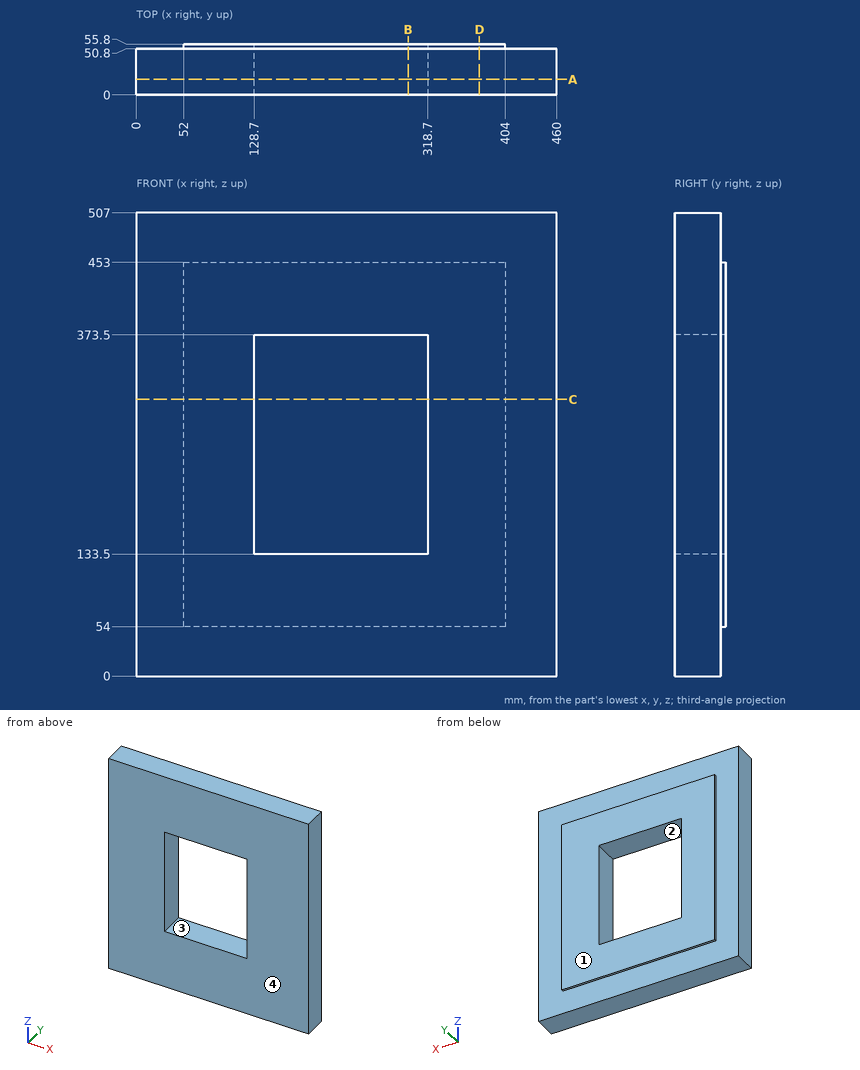
Part print with two shaded views. Sizes in mm from the minimum x, y, z corner. A direction names the side the tool comes from. Coordinates: 2 decimals unless noted, no trailing zeros. Order: outer loops, then holes, each group sorted by start corner. A loop starts at its lowest first (then second) coordinate and runs counter-clockwise, first axis right, second up. Notation, with made-up numbers: (24.25, 24) - (80.25, 24) arc R14 ccw to (80.25, 41) - close; hole circle Ø10 at (-40, 9). An arc over 180 degrees is marked (long way). Write item = value, one per line. Start each with the question number.
1) Flat gauge pins, fed straight in: pin 1 Ø2.5 at (y, z) = (52.5, 316.5) entering from +X; pin 2 Ø4 at (y, z) = (54, 203.5) entering from -X. Where does each tip first touch, or does it go through?
2) Saw through at A-A on y = 17. Write the cut outline in (x, z), then the cut area to 3 significant figures.
3) Two-plate mould, pull along Z, no slides. Class the marked faces 3 and 4: pulls with the +Z half, pulls with the -Z half, needs draft (parallel to the pull), parting line crosses it, or undercut.
4) Wall check: line 1 along X through (y, z) = (12, 138); line 2 along Z through (x, y) = (247.5, 43); line 3 along Y through (x, z) = (437, 138.5). Give the ranges that are in metal, low to high. Write a range as from..to.
5) Saw through at B-B on x = 297.5. Write the cut outline in (y, z), then the cut area to 3 significant figures.
6) Saw through at D-D on x = 375.5. Write the cut outline in (y, z), then the cut area to 3 significant figures.
7) 3-axis set-ups, long thin cutter, end or side, ignore diameter. For the marked faces 1 and 2: which of +Z, -Z, +X, -X, +Y, -Y reach the whole face in a straight line?
8) Saw through at C-C on z = 303. Write the cut outline in (x, y).
From the geometry:
q1.pin_1 = 404
q1.pin_2 = 52
q2.outline = (0, 0) - (460, 0) - (460, 507) - (0, 507) - close; hole (128.7, 133.5) - (318.7, 133.5) - (318.7, 373.5) - (128.7, 373.5) - close
q2.area = 188,000 mm^2
q3.face_3 = undercut
q3.face_4 = needs draft
q4.line_1 = 0..128.7, 318.7..460
q4.line_2 = 0..133.5, 373.5..507
q4.line_3 = 0..50.8
q5.outline = (0, 0) - (50.8, 0) - (50.8, 54) - (55.8, 54) - (55.8, 133.5) - (0, 133.5) - close; (0, 373.5) - (55.8, 373.5) - (55.8, 453) - (50.8, 453) - (50.8, 507) - (0, 507) - close
q5.area = 14,400 mm^2
q6.outline = (0, 0) - (50.8, 0) - (50.8, 54) - (55.8, 54) - (55.8, 453) - (50.8, 453) - (50.8, 507) - (0, 507) - close
q6.area = 27,800 mm^2
q7.face_1 = +Z, -Z, +X, -X, +Y
q7.face_2 = +Y, -Y
q8.outline = (0, 0) - (128.7, 0) - (128.7, 55.8) - (52, 55.8) - (52, 50.8) - (0, 50.8) - close; (318.7, 0) - (460, 0) - (460, 50.8) - (404, 50.8) - (404, 55.8) - (318.7, 55.8) - close
